Autodesk Inventor part; units mm, degrees
ref_plane "YZ Plane" through (0, 0, 0) normal (1, 0, 0) x (0, 1, 0)
ref_plane "XZ Plane" through (0, 0, 0) normal (0, 1, 0) x (-1, 0, 0)
ref_plane "XY Plane" through (0, 0, 0) normal (0, 0, 1) x (1, 0, 0)
ref_plane "Work Plane1" through (49.1494, -37.6525, 49.2967) normal (0, 1, 0) x (-1, 0, 0)
sketch "Sketch2" plane through (49.1494, -37.6525, 49.2967) normal (0, 1, 0) x (-1, 0, 0)
  line L0 (662.4608, -525.6919) -> (646.2945, -509.5274)
  line L1 (143.1429, -6.4305) -> (69.9168, -79.6645)
  line L2 (623.8451, -531.9793) -> (639.991, -548.1234)
  line L3 (104.5272, -12.7179) -> (126.9766, 9.734)
  line L4 (646.2945, -509.5274) -> (662.4608, -525.6919)
  line L5 (662.4608, -525.6919) -> (639.991, -548.1234)
  line L6 (639.991, -548.1234) -> (623.8451, -531.9793)
  line L7 (623.8451, -531.9793) -> (646.2945, -509.5274)
  point P0 (49.1494, -49.2967)
  point P1 (69.9168, -79.6645)
extrude "Extrusion2" add sketch "Sketch2" along normal blind 44.45
sketch "Sketch3" plane through (49.1494, 6.7975, 49.2967) normal (0, 1, 0) x (1, 0, 0)
  circle A0 centre (-647.1931, 521.2017) radius 2.4765
  circle A1 centre (-635.5195, 532.8766) radius 2.4765
  point P0 (-49.1494, 49.2967)
hole "Hole1" at (-586.3701, 6.7975, -483.58) at (-598.0438, 6.7975, -471.905) direction (0, -1, 0) diameter 7.112 depth 10.414
sketch "Sketch4" plane through (49.1494, -37.6525, 49.2967) normal (0, -1, 0) x (1, 0, 0)
  circle A0 centre (-647.1931, -521.2017) radius 3.556
  circle A1 centre (-635.5195, -532.8766) radius 3.556
  point P0 (-49.1494, -49.2967)
extrude "Extrusion3" cut sketch "Sketch4" against normal blind 10.414
fillet "Fillet1" radius 3.175 2 edges at (-590.8417, -15.4275, -498.8268) (-613.3114, -15.4275, -476.3953)
properties part number "Standoff"
Design review of the part built by this model. Coordinates are the model's own, in mm. A direction names the side the tool comes from. Coordinates: 2 decimals unless noted, no trailing zeros. Order: outer loops, then holes, each group sorted by start corner. A loop starts at its lowest first (then second) coordinate and runs counter-clockwise, first axis right, second up.
Item 1: The part is to be moulded in two halves that separate along Z. For faces 1 (the cylindrical face through (-611.994, -15.116, -476.43)), 2 (the flat face through (-586, -3.616, -484)), 3 (the flat face through (-593, 6.798, -479)), say which applies: pulls with the +Z half, pulls with the -Z half, needs draft (parallel to the pull), parting line crosses it, or undercut.
Item 2: For faces 4 (the flat face through (-598, -27.238, -472)), 5 (the flat face through (-598, -3.616, -472)), 6 (the flat face through (-585.763, -15.739, -471.614)), list the 3-axis set-ups (+Z, -Z, +X, -X, +Y, -Y) from which the entire face can be reached by the end or side of a thin tool; tool diameter is ignored.
Item 3: For line 1 (X direction, y = -31.5, z = -470); line 2 (Z direction, x = -585.5, y = 3.5); line 3 (Z direction, x = -608.5, y = -27), list the stretches that pass through material, from the lowest coordinate up.
Item 4: Take a section at C-C, the plane y = -17. Write out the cut boundary in (x, z) (3 decimals).
Item 5: Take a section at B-B, the plane z = -470. Write out the cut boundary in (x, y).
Item 6: For pin 1 Ø5.5 at (x, z) = (-586.37, -483.58) entering from +Y; pin 2 Ø1.5 at (y, z) = (-4, -481.5) entering from +X; pin 3 Ø2 at (y, z) = (-8, -468) entering from -X, all flat-tipped, find the tip position at first contact; note any pin that passes through.
Item 7: Take a section at A-A, the plane y = -28. Write out the cut boundary in (x, z) (3 decimals).
Item 8: Take a section at D-D, the plane x = -604. Write out the cut boundary in (y, z), then the cut area to 3 significant figures.
The answers:
1. face 1: parting line crosses it
1. face 2: undercut
1. face 3: needs draft
2. face 4: -Y
2. face 5: +Y
2. face 6: +Z, +X, +Y, -Y
3. line 1: x = -606.92 to -601.05, -595.04 to -587.38
3. line 2: z = -493.49 to -487.03, -480.13 to -471.88
3. line 3: z = -481.2 to -471.58
4. outline: (-611.064, -474.148) arc R3.175 ccw to (-611.062, -478.64) - (-593.087, -496.586) arc R3.175 ccw to (-588.598, -496.584) - (-574.696, -482.683) - (-597.145, -460.231) - close
5. outline: (-606.92, -37.65) - (-601.05, -37.65) - (-601.05, -27.24) - (-595.04, -27.24) - (-595.04, -37.65) - (-587.38, -37.65) - (-587.38, 6.8) - (-595.04, 6.8) - (-595.04, -3.62) - (-601.05, -3.62) - (-601.05, 6.8) - (-606.92, 6.8) - close
6. pin 1: stops at y = -3.62
6. pin 2: stops at x = -575.13
6. pin 3: stops at x = -605.92
7. outline: (-611.064, -474.148) arc R3.175 ccw to (-611.062, -478.64) - (-593.087, -496.586) arc R3.175 ccw to (-588.598, -496.584) - (-574.696, -482.683) - (-597.145, -460.231) - close; hole circle Ø7.112 at (-598.044, -471.905); hole circle Ø7.112 at (-586.37, -483.58)
8. outline: (-37.65, -485.69) - (6.8, -485.69) - (6.8, -467.08) - (-37.65, -467.08) - close
8. area: 827 mm2
